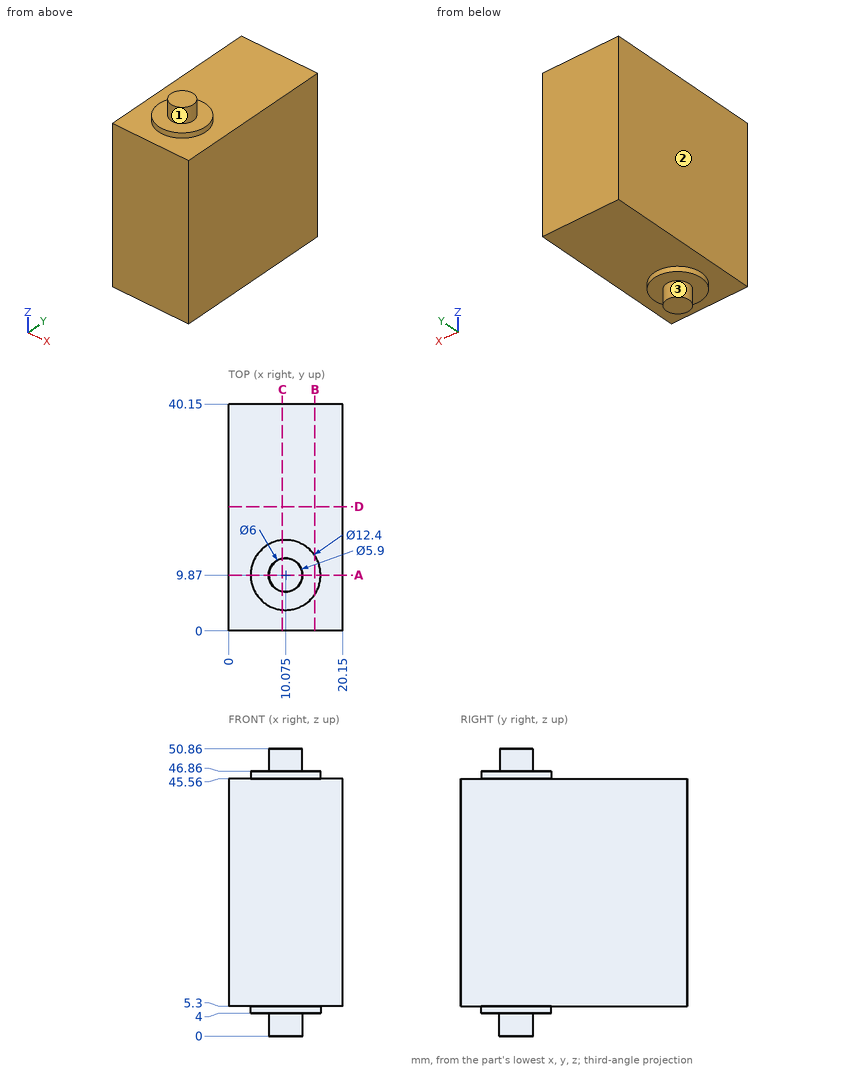
Print and shaded views of the part. All mm, measured from the part's lowest x, y and z. A direction names the side the tool comes from. Coordinates: 2 decimals unless noted, no trailing zeros. Loops run counter-clockwise (first coordinate to the right, second up) from the corner with the lowest first, then second, coordinate; pieces in that order, holes last. Notation, with made-up numbers: (77.5, 8) - (82.5, 8) arc R18 cw to (82.5, 30) - close; hole circle Ø6 at (-26, 3). An arc over 180 degrees is marked (long way). Write item = value, one per line. Start each with the question number.
Item 1: Saw through at B-B, the plane x = 15.25. List the corners of the cut face in (y, z).
Item 2: Saw through at A-A, the plane y = 9.87. List the corners of the cut face in (x, z) (3 decimals), then the cut area to 3 significant figures.
Item 3: Saw through at C-C, the plane x = 9.5. List the corners of the cut face in (y, z).
Item 4: 3-axis set-ups, long thin cutter, end or side, ignore diameter. For the marked faces 1, 2 and 3: which of +Z, -Z, +X, -X, +Y, -Y reach the whole face in a straight line?
Item 5: Wall check: probe 1 along Z at (x, y) = (17, 3); probe 2 along Z at (x, y) = (7.75, 13.5). Give the ranges that are in metal, low to high. Write a range as [from, to].
Item 6: Drop flat-ended pins along their axis: pin 1 Ø1 at (x, y) = (11.5, 19.5) entering from +Z; pin 2 Ø6 at (x, y) = (9, 17) entering from +Z. Give the stop position or say it passes through.
Item 7: Saw through at D-D, the plane y = 22. List the corners of the cut face in (x, z), then the cut area to 3 significant figures.
Answers:
q1.outline = (0, 5.3) - (6.46, 5.3) - (6.46, 4) - (13.28, 4) - (13.28, 5.3) - (40.15, 5.3) - (40.15, 45.56) - (13.28, 45.56) - (13.28, 46.86) - (6.46, 46.86) - (6.46, 45.56) - (0, 45.56) - close
q2.outline = (0, 5.3) - (3.875, 5.3) - (3.875, 4) - (7.075, 4) - (7.075, 0) - (13.075, 0) - (13.075, 4) - (16.275, 4) - (16.275, 5.3) - (20.15, 5.3) - (20.15, 45.56) - (16.275, 45.56) - (16.275, 46.86) - (13.025, 46.86) - (13.025, 50.86) - (7.125, 50.86) - (7.125, 46.86) - (3.875, 46.86) - (3.875, 45.56) - (0, 45.56) - close
q2.area = 891 mm2
q3.outline = (0, 5.3) - (3.7, 5.3) - (3.7, 4) - (6.93, 4) - (6.93, 0) - (12.81, 0) - (12.81, 4) - (16.04, 4) - (16.04, 5.3) - (40.15, 5.3) - (40.15, 45.56) - (16.04, 45.56) - (16.04, 46.86) - (12.76, 46.86) - (12.76, 50.86) - (6.98, 50.86) - (6.98, 46.86) - (3.7, 46.86) - (3.7, 45.56) - (0, 45.56) - close
q4.face_1 = +Z
q4.face_2 = +Z, -Z, -X, +Y, -Y
q4.face_3 = -Z
q5.probe_1 = [5.3, 45.56]
q5.probe_2 = [4, 46.86]
q6.pin_1 = 45.56
q6.pin_2 = 46.86
q7.outline = (0, 5.3) - (20.15, 5.3) - (20.15, 45.56) - (0, 45.56) - close
q7.area = 811 mm2
